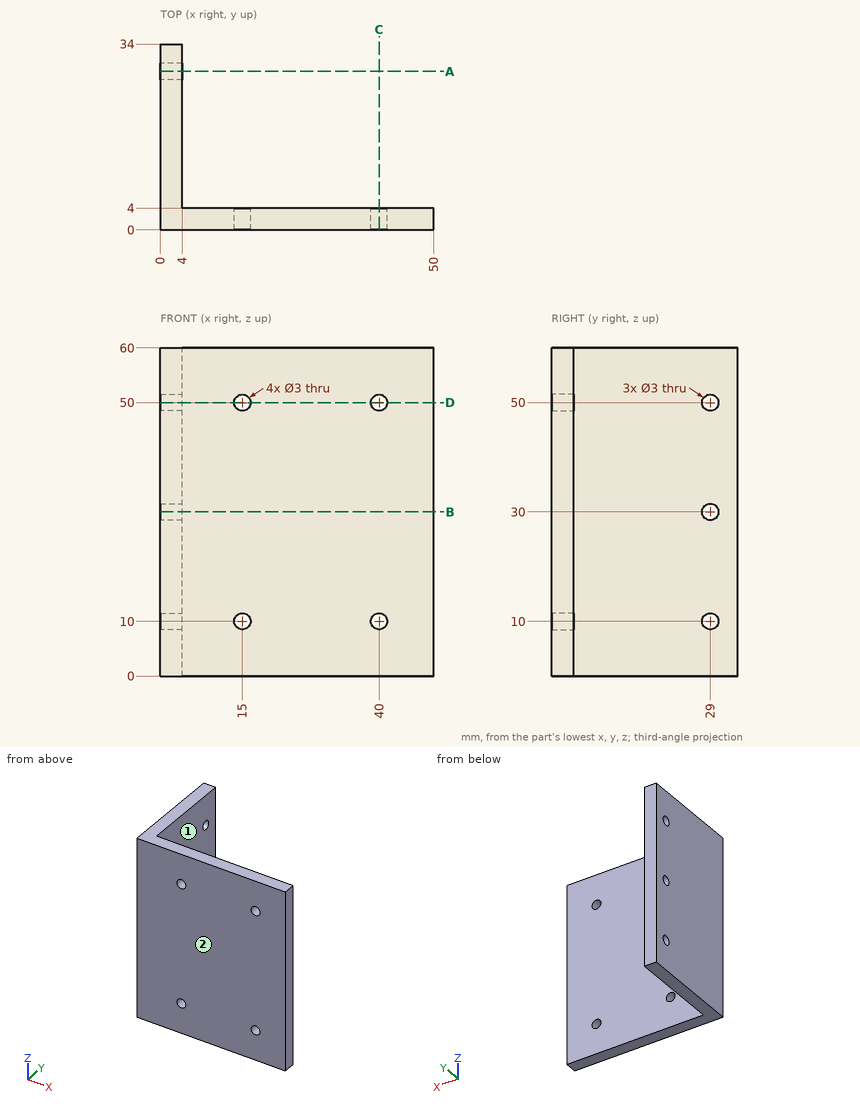
Input: dimensioned drawing with shaded views. Units: mm. Origin: part minimum x, y, z. A direction names the side the tool comes from. Round coordinates to 2 decimals unless told otherwise and drop trailing zeros. Order: outer loops, then holes, each group sorted by start corner. A loop starts at its lowest first (then second) coordinate and runs counter-clockwise, first axis right, second up.
1. Cut plane C-C, the plane x = 40. Output: boundary loops of the cut face in (y, z).
The answers:
outline: (0, 0) - (4, 0) - (4, 8.5) - (0, 8.5) - close; (0, 11.5) - (4, 11.5) - (4, 48.5) - (0, 48.5) - close; (0, 51.5) - (4, 51.5) - (4, 60) - (0, 60) - close
2. Cut plane D-D, the plane z = 50. Output: boundary loops of the cut face in (x, y), then the cut area to 3 significant figures.
The answers:
outline: (0, 0) - (13.5, 0) - (13.5, 4) - (4, 4) - (4, 27.5) - (0, 27.5) - close; (0, 30.5) - (4, 30.5) - (4, 34) - (0, 34) - close; (16.5, 0) - (38.5, 0) - (38.5, 4) - (16.5, 4) - close; (41.5, 0) - (50, 0) - (50, 4) - (41.5, 4) - close
area: 284 mm2
3. Cut plane B-B, the plane z = 30. Output: boundary loops of the cut face in (x, y), then the cut area to 3 significant figures.
The answers:
outline: (0, 0) - (50, 0) - (50, 4) - (4, 4) - (4, 27.5) - (0, 27.5) - close; (0, 30.5) - (4, 30.5) - (4, 34) - (0, 34) - close
area: 308 mm2
4. Cut plane A-A, the plane y = 29. Output: boundary loops of the cut face in (x, z).
The answers:
outline: (0, 0) - (4, 0) - (4, 8.5) - (0, 8.5) - close; (0, 11.5) - (4, 11.5) - (4, 28.5) - (0, 28.5) - close; (0, 31.5) - (4, 31.5) - (4, 48.5) - (0, 48.5) - close; (0, 51.5) - (4, 51.5) - (4, 60) - (0, 60) - close
5. Set-up query: the marked faces 1 and 2. Return all of +Z, -Z, +X, -X, +Y, -Y with unobstructed straight access to the full face (end or side cutting, diameter ignored); none if empty.
The answers:
face 1: +Z, -Z, +X, +Y
face 2: +Z, -Z, +X, -X, -Y
6. Pin query (flat end, axial travel): P1, Ø23, axis at x = 37.5, z = 20, coming from the +Y side; P2, Ø2.5, axis at x = 40, z = 50, coming from the -Y side. Return the tip coordinate at first contact, or that it passes through.
The answers:
P1: stops at y = 4
P2: passes through
7. Material intervals for line 1 (X direction, y = 2.5, z = 10); line 2 (Y direction, x = 2, z = 30); line 3 (Y direction, x = 41, z = 43), sorted ascending.
The answers:
line 1: x = 0 to 13.5, 16.5 to 38.5, 41.5 to 50
line 2: y = 0 to 27.5, 30.5 to 34
line 3: y = 0 to 4
